Input: part model. Units: mm. Frame: model coordinates. Face numbers are marked on the shaded views. Give positions to 0.01 mm unless a question says otherwise; leave off trailing zeros. Order: outer loops, then holes, each group sorted by start corner. A loop starts at its lowest first (then second) coordinate and runs counter-clockwise, first axis right, second up. Notation, with made-up numbers: (65, -23.5) - (84, -23.5) arc R14 cw to (84, 0.5) - close; hole circle Ø2 at (82.25, 80.25). An arc over 180 degrees is marked (long way). Use a Markdown table: item, result.
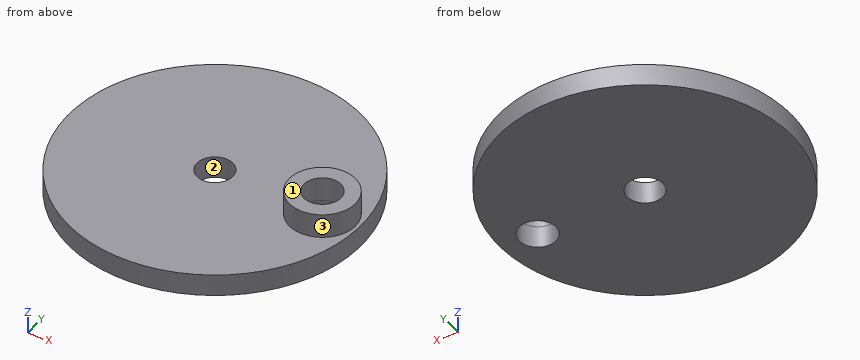
from build123d import *

# Parameters (mm, degrees)
SKETCH1_R               = 20
BOSS_EXTRUDE1_DEPTH     = 3
CUT_EXTRUDE3_START      = 3
SKETCH2_R               = 2.525
CUT_EXTRUDE3_DEPTH      = 4
CUT_EXTRUDE3_DEPTH_BACK = 4
BOSS_EXTRUDE2_START     = 3
SKETCH3_R               = 4.525
SKETCH3_R_2             = 2.525
BOSS_EXTRUDE2_DEPTH     = 3.3
SKETCH4_R               = 2.45
CUT_EXTRUDE4_DEPTH      = 7.3


with BuildPart() as part:
    # Sketch1 → Boss-Extrude1 (new body)
    with BuildSketch(Plane.XY):
        Circle(SKETCH1_R)
    extrude(amount=BOSS_EXTRUDE1_DEPTH)

    # Sketch2 → Cut-Extrude3 (cut, two sides)
    with BuildSketch(Plane.XY.offset(CUT_EXTRUDE3_START)) as cut_extrude3_sk:
        with Locations((15, 0)):
            Circle(SKETCH2_R)
    extrude(amount=CUT_EXTRUDE3_DEPTH, mode=Mode.SUBTRACT)
    extrude(cut_extrude3_sk.sketch, amount=-CUT_EXTRUDE3_DEPTH_BACK, mode=Mode.SUBTRACT)

    # Sketch3 → Boss-Extrude2 (add)
    with BuildSketch(Plane.XY.offset(BOSS_EXTRUDE2_START)):
        with Locations((15, 0)):
            Circle(SKETCH3_R)
        with Locations((15, 0)):
            Circle(SKETCH3_R_2, mode=Mode.SUBTRACT)
    extrude(amount=BOSS_EXTRUDE2_DEPTH)

    # Sketch4 → Cut-Extrude4 (cut, through all)
    with BuildSketch(Plane.XY):
        Circle(SKETCH4_R)
    extrude(amount=CUT_EXTRUDE4_DEPTH, mode=Mode.SUBTRACT)


solid = part.part
1. Section query B-B (y = 0). Return loops of the section in (x, z) (3 decimals), then the cut area to 3 significant figures.
Response:
| item | result |
|---|---|
| outline | (-20, 0) - (-2.45, 0) - (-2.45, 3) - (-20, 3) - close; (2.45, 0) - (12.475, 0) - (12.475, 6.3) - (10.475, 6.3) - (10.475, 3) - (2.45, 3) - close; (17.525, 0) - (20, 0) - (20, 3) - (19.525, 3) - (19.525, 6.3) - (17.525, 6.3) - close |
| area | 103 mm^2 |
2. Material intervals for line 1 along Y through (x, z) = (15, 4.55) (3 decimals); line 2 along Z through (x, y) = (13, -13); line 3 along Y through (x, z) = (0, 0.9), sorted ascending.
Response:
| item | result |
|---|---|
| line 1 | y = -4.525 to -2.525, 2.525 to 4.525 |
| line 2 | z = 0 to 3 |
| line 3 | y = -20 to -2.45, 2.45 to 20 |
3. Section query A-A (x = 0). Return loops of the section in (y, z).
Response:
| item | result |
|---|---|
| outline | (-20, 0) - (-2.45, 0) - (-2.45, 3) - (-20, 3) - close; (2.45, 0) - (20, 0) - (20, 3) - (2.45, 3) - close |
4. Mould query, pull axis X, two halves, no side actions, for the marked faces 1, 2 and 3. Classes: pulls with the +X half, pulls with the -X half, needs draft (parallel to the pull), parting line crosses it, or undercut.
Response:
| item | result |
|---|---|
| face 1 | needs draft |
| face 2 | undercut |
| face 3 | parting line crosses it |
5. Section query D-D (z = 0.75). Return loops of the section in (x, y) (3 decimals), then the cut area to 3 significant figures.
Response:
| item | result |
|---|---|
| outline | circle Ø40 at (0, 0); hole circle Ø4.9 at (0, 0); hole circle Ø5.05 at (15, 0) |
| area | 1,220 mm^2 |
6. Pin query (flat end, axial travel): pin 1 (2 mm diameter, centred on y = -8.5, z = 2.5, fed in from -X); pin 2 (8 mm diameter, centred on x = -1.5, y = 13, fed in from +Z); pin 3 (1.5 mm diameter, centred on y = 14, z = 4.5, fed in from -X); pin 4 (1.5 mm diameter, centred on x = 12.5, z = 0.5, fed in from -Y). Return the tip coordinate at first contact, or that it passes through.
Response:
| item | result |
|---|---|
| pin 1 | stops at x = -18.54 |
| pin 2 | stops at z = 3 |
| pin 3 | passes through |
| pin 4 | stops at y = -16.18 |
7. Section query C-C (z = 5.75). Return loops of the section in (x, y) (3 decimals), then the cut area to 3 significant figures.
Response:
| item | result |
|---|---|
| outline | circle Ø9.05 at (15, 0); hole circle Ø5.05 at (15, 0) |
| area | 44.3 mm^2 |
